Can you work these out from the drawing? Everything is in mm from the part's minimum corner. Give positions to 0.01 mm unless a question says otherwise; leave off trailing zeros. Order: outer loops, then holes, each group sorted by start corner. A loop starts at its lowest first (then second) coordinate and runs counter-clockwise, first axis right, second up. Notation, with made-up numbers: (-10, 4) - (25, 4) arc R13 cw to (25, 19) - close; hole circle Ø2 at (19, 21.5). An arc over 180 degrees is marked (long way). Answer as a JSON object with one key per item and string values.
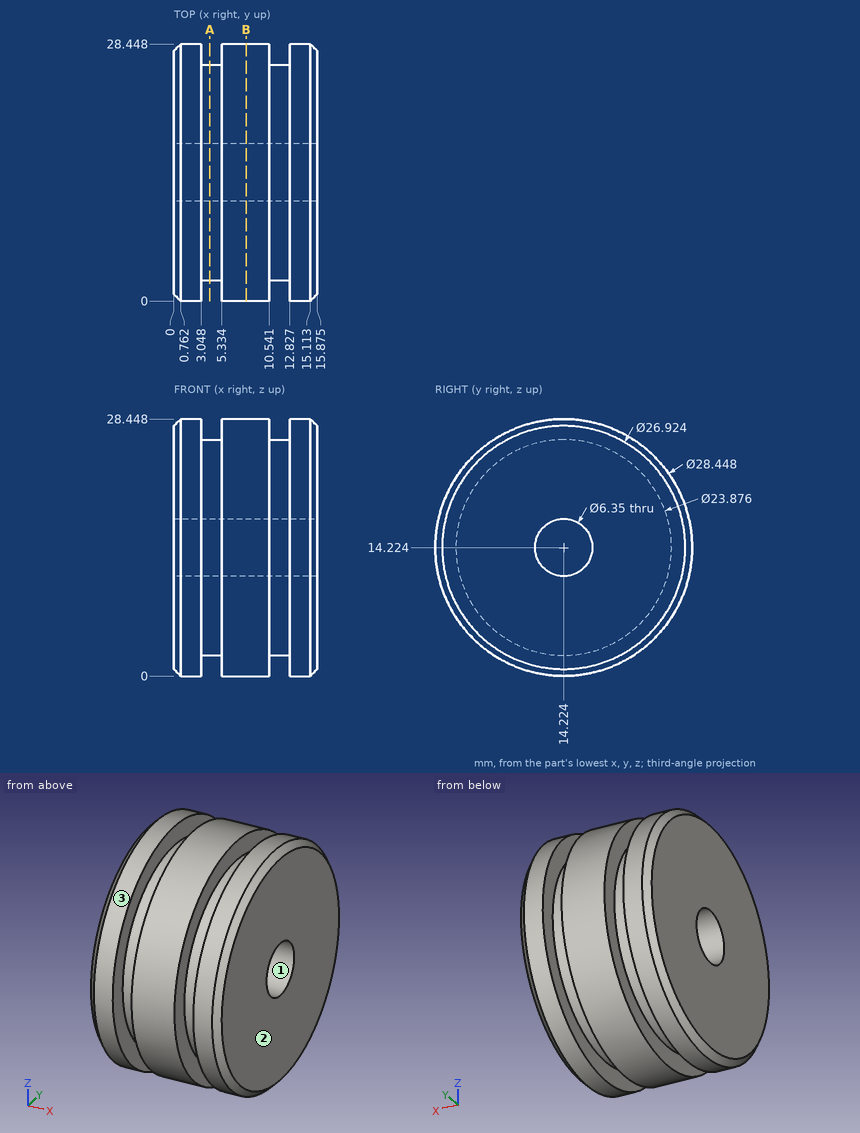
Q1. If we section it at B-B, the plane x = 8: Please give me the cut outline in (y, z) (3 decimals), then the cut area to 3 significant figures.
Recorded:
{"outline": "circle Ø28.448 at (14.224, 14.224); hole circle Ø6.35 at (14.224, 14.224)", "area": "604 mm^2"}
Q2. We'd pull the mould along Y, two halves only. Please class the marked faces 1, 2 and 3: released by +Y, released by -Y, zero draft, split by the parting line, or undercut.
Recorded:
{"face 1": "undercut", "face 2": "zero draft", "face 3": "split by the parting line"}
Q3. I need wall thicknesses on L1, parallel to X at y = 23.75, z = 6.75 (3 decimals); L2, parallel to Y at x = 10, z = 14.25; L3, parallel to Y at x = 8.5, z = 14. Which ranges of each line are inside material? Lowest first, please.
Recorded:
{"L1": "x = 0 to 3.048, 5.334 to 10.541, 12.827 to 15.875", "L2": "y = 0 to 11.05, 17.4 to 28.45", "L3": "y = 0 to 11.06, 17.39 to 28.45"}
Q4. If we section it at A-A, the plane x = 4: Please give me the cut outline in (y, z) (3 decimals), then the cut area to 3 significant figures.
Recorded:
{"outline": "circle Ø23.876 at (14.224, 14.224); hole circle Ø6.35 at (14.224, 14.224)", "area": "416 mm^2"}
Q5. I'm going to push flat-ended pins straight in: pin 1 Ø8 at (x, z) = (10, 3.5) entering from +Y; pin 2 Ø2 at (x, y) = (8.5, 18.5) entering from -Z; pin 3 Ø4 at (y, z) = (14.224, 14.224) entering from -X; pin 4 Ø3 at (x, z) = (4, 20) entering from -Y. Where does each tip first touch, or does it pass through?
Recorded:
{"pin 1": "stops at y = 26.76", "pin 2": "stops at z = 0.38", "pin 3": "passes through", "pin 4": "stops at y = 0.77"}
